Check sheet for the drawn part. Datum: minimum x, y, z corner. Units: mm. Give positions to 0.01 mm unless a question says otherwise; leave off trailing zeros. Write each loop counter-clockwise with the first axis right and the second up, starting at its lowest first coordinate (ties: lowest second). Pieces come first, ordered by that corner, then holes. Notation, with made-up numbers: (11.5, 80) -> (28.5, 80) arc R24 ccw to (28.5, 115) -> close; hole circle Ø4 at (71, -15.5). An arc over 180 degrees is marked (long way). Write item = value, one per line. Start each with the question number.
1. Thickness scan on line 1 along Y through (x, z) = (37.5, 0.85); line 2 along Y through (x, z) = (55, 0.8) (1 decimal); line 3 along X through (y, z) = (50, 1.2). Record the ranges inside material, lowest first.
2. Cross-section at B-B, the plane x = 38.5. Record the cut outline in (y, z).
3. Cross-section at C-C, the plane z = 1.05. State how many separate pieces and enclosed holes the cut face has, plus the area to 3 significant figures.
4. Cross-section at A-A, the plane y = 105. Record the cut outline in (x, z).
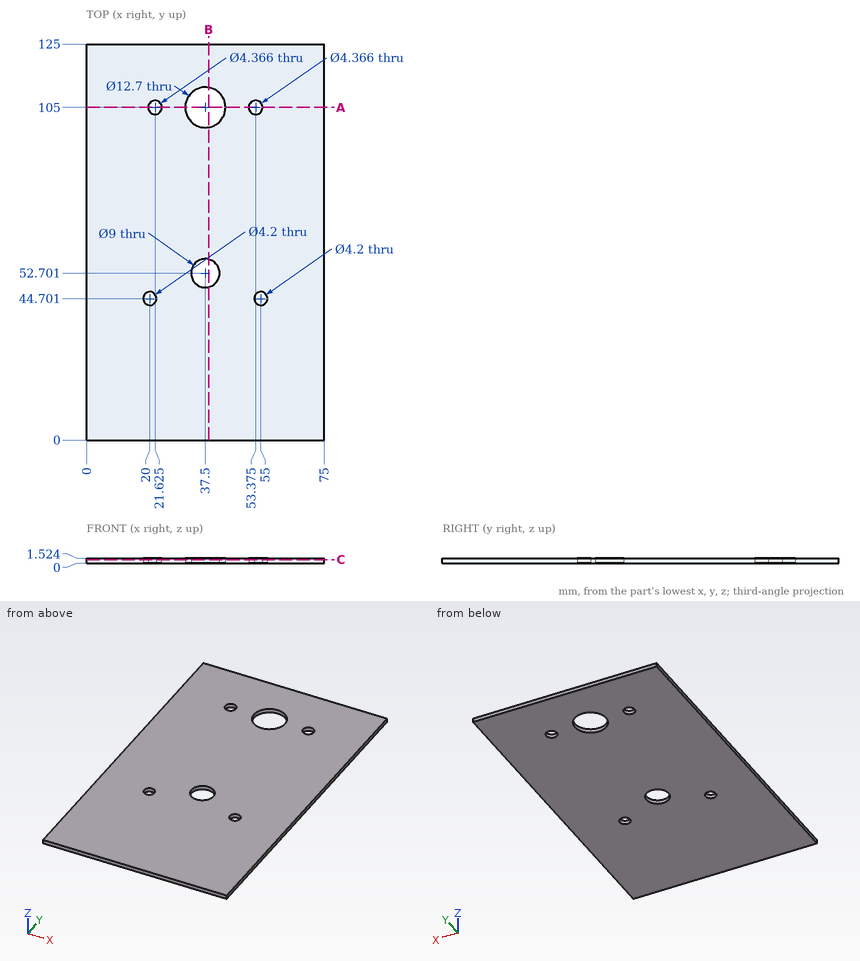
Answers:
q1.line_1 = 0 to 48.2, 57.2 to 98.65, 111.35 to 125
q1.line_2 = 0 to 42.6, 46.8 to 103.5, 106.5 to 125
q1.line_3 = 0 to 33.9, 41.1 to 75
q2.outline = (0, 0) -> (48.31, 0) -> (48.31, 1.52) -> (0, 1.52) -> close; (57.09, 0) -> (98.73, 0) -> (98.73, 1.52) -> (57.09, 1.52) -> close; (111.27, 0) -> (125, 0) -> (125, 1.52) -> (111.27, 1.52) -> close
q3.separate_pieces = 1
q3.enclosed_holes = 6
q3.area = 9,130 mm^2
q4.outline = (0, 0) -> (19.44, 0) -> (19.44, 1.52) -> (0, 1.52) -> close; (23.81, 0) -> (31.15, 0) -> (31.15, 1.52) -> (23.81, 1.52) -> close; (43.85, 0) -> (51.19, 0) -> (51.19, 1.52) -> (43.85, 1.52) -> close; (55.56, 0) -> (75, 0) -> (75, 1.52) -> (55.56, 1.52) -> close
